from build123d import *

# Parameters (mm, degrees)
SKETCH_1_W          = 80
SKETCH_1_H          = 80
EXTRUDE_1_DEPTH     = 10.5
SKETCH_3_R          = 10.35
SKETCH_3_R_2        = 1.65
CUT_EXTRUDE_1_DEPTH = 62.116691664
SKETCH_2_W          = 50
SKETCH_2_H          = 30
CUT_EXTRUDE_2_DEPTH = 5.5
SKETCH_6_W          = 45.255083204
SKETCH_6_H          = 30
CUT_EXTRUDE_3_DEPTH = 7
SKETCH_7_R          = 1.65
CUT_EXTRUDE_4_DEPTH = 62.116691664
FILLET_1_R          = 8
FILLET_2_R          = 8
FILLET_3_R          = 8
FILLET_4_R          = 8
SKETCH_9_R          = 1.65
CUT_EXTRUDE_5_DEPTH = 62.116691664


with BuildPart() as part:
    # 草图1 → 凸台-拉伸1 (new body)
    with BuildSketch(Plane.XY):
        with Locations((-5, 0)):
            Rectangle(SKETCH_1_W, SKETCH_1_H)
    extrude(amount=EXTRUDE_1_DEPTH)

    # 草图3 → 切除-拉伸1 (cut, through all)
    with BuildSketch(Plane.XY.offset(10.5)):
        with Locations((10.25, 15)):
            Circle(SKETCH_3_R)
        with Locations((-19.95, 15)):
            Circle(SKETCH_3_R_2)
        with Locations((-9.86238383, 35)):
            Circle(SKETCH_3_R_2)
        with Locations((0.16238383, 35)):
            Circle(SKETCH_3_R_2)
    extrude(amount=-CUT_EXTRUDE_1_DEPTH, mode=Mode.SUBTRACT)

    # 草图2 → 切除-拉伸2 (cut)
    with BuildSketch(Plane.XY.offset(10.5)):
        with Locations((0, 15)):
            Rectangle(SKETCH_2_W, SKETCH_2_H)
    extrude(amount=-CUT_EXTRUDE_2_DEPTH, mode=Mode.SUBTRACT)

    # 草图6 → 切除-拉伸3 (cut)
    with BuildSketch(Plane.XY.offset(10.5)):
        with Locations((-0.553390963, 15)):
            Rectangle(SKETCH_6_W, SKETCH_6_H)
    extrude(amount=-CUT_EXTRUDE_3_DEPTH, mode=Mode.SUBTRACT)

    # 草图7 → 切除-拉伸4 (cut, through all)
    with BuildSketch(Plane.XY.offset(10.5)):
        with Locations((-5, -12.75)):
            Circle(SKETCH_7_R)
        with Locations((2.25, -20)):
            Circle(SKETCH_7_R)
        with Locations((-5, -27.25)):
            Circle(SKETCH_7_R)
        with Locations((-12.25, -20)):
            Circle(SKETCH_7_R)
    extrude(amount=-CUT_EXTRUDE_4_DEPTH, mode=Mode.SUBTRACT)

    # 圆角1
    fillet_1_edges = [part.edges().sort_by_distance(p)[0] for p in [
        (-45, -40, 5.25),
    ]]
    fillet(fillet_1_edges, radius=FILLET_1_R)

    # 圆角2
    fillet_2_edges = [part.edges().sort_by_distance(p)[0] for p in [
        (35, -40, 5.25),
    ]]
    fillet(fillet_2_edges, radius=FILLET_2_R)

    # 圆角3
    fillet_3_edges = [part.edges().sort_by_distance(p)[0] for p in [
        (35, 40, 5.25),
    ]]
    fillet(fillet_3_edges, radius=FILLET_3_R)

    # 圆角4
    fillet_4_edges = [part.edges().sort_by_distance(p)[0] for p in [
        (-45, 40, 5.25),
    ]]
    fillet(fillet_4_edges, radius=FILLET_4_R)

    # 草图9 → 切除-拉伸5 (cut, through all)
    with BuildSketch(Plane(origin=(0, 0, 0), x_dir=(-1, 0, 0), z_dir=(0, 0, -1))):
        with Locations((-29.828427125, -34.828427125)):
            Circle(SKETCH_9_R)
        with Locations((39.828427125, -34.828427125)):
            Circle(SKETCH_9_R)
        with Locations((-29.828427125, -5)):
            Circle(SKETCH_9_R)
        with Locations((39.828427125, -5)):
            Circle(SKETCH_9_R)
    extrude(amount=-CUT_EXTRUDE_5_DEPTH, mode=Mode.SUBTRACT)


solid = part.part
Model file for the job. Use its own axes, mm. A direction names the side the tool comes from. Coordinates: 2 decimals unless noted, no trailing zeros. Write each loop counter-clockwise with the first axis right and the second up, starting at its lowest first coordinate (ties: lowest second). Pieces come first, ordered by that corner, then holes. Notation, with made-up numbers: (36, 23) -> (55, 23) arc R9 ccw to (55, 29) -> close; hole circle Ø6 at (12.25, 23). An arc over 180 degrees is marked (long way). One line per item, written item: value. Start each with the question number.
1) Pull direction Y, two halves, no side cores. Call faces 1 (the face through (-6.31, -13.75, 5.32)), 2 (the face through (-42.594, 37.719, 5.324)), 3 (the face through (-6, -8, 10.5)), 4 (the face through (25, 15, 8)): +Y half, -Y half, draft (parallel to the pull), parting line (faces both ways), or undercut.
2) Which spindle directions (+Z, -Z, +X, -X, +Y, -Y) get a long thin tool onto all of the face, cutting with end or side? Do faces 5 (the face through (32.719, 37.594, 5.324)), 6 (the face through (-24, 15, 5)). Say none if no direction does.
3) Slice it at B-B on y = 15. Write the cut outline in (x, z).
4) Flat gauge pin, fed straight in: pin 1 Ø12.5 at (x, y) = (10.25, 15) entering from +Z. Where does the tip first touch, or does it go through?
5) Slice it at D-D on z = 8. Count the separate pieces of the cut face and the enclosed holes in it, then the cut area to 3 significant figures.
6) Probe probe 1 along Y at (x, z) = (-3, 10.25); probe 2 along Y at (x, z) = (-38.5, 4.5); probe 3 along Y at (x, z) = (-6, 6.5). List the from-to ranges inside material, lowest first.
7) Slice it at A-A on x = -5. Write the cut outline in (y, z).
8) Slice it at C-C on x = 10.25. Write the cut outline in (y, z).
Answers follow:
1. face 1: undercut
1. face 2: +Y half
1. face 3: draft
1. face 4: undercut
2. face 5: +Z, -Z, +X, +Y
2. face 6: +Z
3. outline: (-45, 0) -> (-21.6, 0) -> (-21.6, 3.5) -> (-23.18, 3.5) -> (-23.18, 5) -> (-25, 5) -> (-25, 10.5) -> (-45, 10.5) -> close; (-18.3, 0) -> (-0.1, 0) -> (-0.1, 3.5) -> (-18.3, 3.5) -> close; (20.6, 0) -> (35, 0) -> (35, 10.5) -> (25, 10.5) -> (25, 5) -> (22.07, 5) -> (22.07, 3.5) -> (20.6, 3.5) -> close
4. pin 1: through
5. separate pieces: 1
5. enclosed holes: 11
5. area: 4,760 mm2
6. probe 1: -40 to 0, 30 to 40
6. probe 2: -39.86 to -35.81, -33.85 to -5.98, -4.02 to 39.86
6. probe 3: -40 to -28.56, -25.94 to -14.06, -11.44 to 0, 30 to 40
7. outline: (-40, 0) -> (-28.9, 0) -> (-28.9, 10.5) -> (-40, 10.5) -> close; (-25.6, 0) -> (-14.4, 0) -> (-14.4, 10.5) -> (-25.6, 10.5) -> close; (-11.1, 0) -> (40, 0) -> (40, 10.5) -> (30, 10.5) -> (30, 3.5) -> (0, 3.5) -> (0, 10.5) -> (-11.1, 10.5) -> close
8. outline: (-40, 0) -> (4.65, 0) -> (4.65, 3.5) -> (0, 3.5) -> (0, 10.5) -> (-40, 10.5) -> close; (25.35, 0) -> (40, 0) -> (40, 10.5) -> (30, 10.5) -> (30, 3.5) -> (25.35, 3.5) -> close
